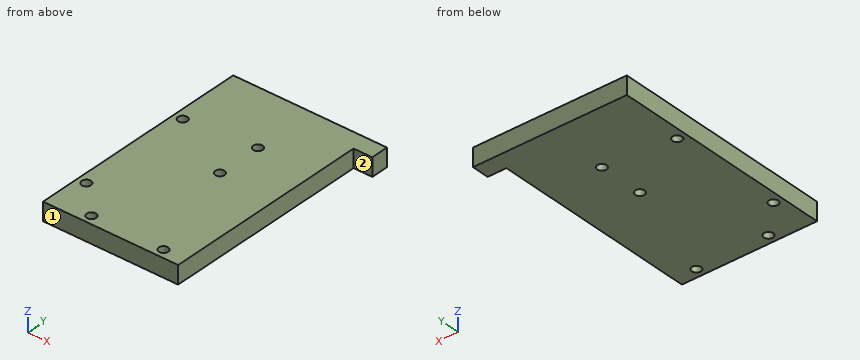
```python
from build123d import *

# Parameters (mm, degrees)
SZKIC1_W                    = 51
SZKIC1_H                    = 75
DODANIE_WYCI_GNI_CIE1_DEPTH = 6
SZKIC3_R                    = 1.55
WYTNIJ_WYCI_GNI_CIE1_DEPTH  = 99.368039697
SZKIC5_R                    = 1.55
WYTNIJ_WYCI_GNI_CIE2_DEPTH  = 6
SZKIC6_W                    = 6.4
SZKIC6_H                    = 69.4
WYTNIJ_WYCI_GNI_CIE3_DEPTH  = 10


with BuildPart() as part:
    # Szkic1 → Dodanie-wyciągnięcie1 (new body)
    with BuildSketch(Plane.XY):
        with Locations((29.991181586, 43.5)):
            Rectangle(SZKIC1_W, SZKIC1_H)
    extrude(amount=DODANIE_WYCI_GNI_CIE1_DEPTH)

    # Szkic3 → Wytnij-wyciągnięcie1 (cut, through all)
    with BuildSketch(Plane(origin=(0, 0, 0), x_dir=(-1, 0, 0), z_dir=(0, 0, -1))):
        with Locations((-18.041181586, 9)):
            Circle(SZKIC3_R)
        with Locations((-41.941181586, 9)):
            Circle(SZKIC3_R)
        with Locations((-7.491181586, 19.55)):
            Circle(SZKIC3_R)
        with Locations((-7.491181586, 57.55)):
            Circle(SZKIC3_R)
    extrude(amount=-WYTNIJ_WYCI_GNI_CIE1_DEPTH, mode=Mode.SUBTRACT)

    # Szkic5 → Wytnij-wyciągnięcie2 (cut)
    with BuildSketch(Plane(origin=(0, 0, 0), x_dir=(-1, 0, 0), z_dir=(0, 0, -1))):
        with Locations((-30.491181586, 59.871958533)):
            Circle(SZKIC5_R)
        with Locations((-30.491181586, 44.871958533)):
            Circle(SZKIC5_R)
    extrude(amount=-WYTNIJ_WYCI_GNI_CIE2_DEPTH, mode=Mode.SUBTRACT)

    # Szkic6 → Wytnij-wyciągnięcie3 (cut)
    with BuildSketch(Plane(origin=(0, 0, 0), x_dir=(-1, 0, 0), z_dir=(0, 0, -1))):
        with Locations((-52.491181586, 40.5)):
            Rectangle(SZKIC6_W, SZKIC6_H)
    extrude(amount=-WYTNIJ_WYCI_GNI_CIE3_DEPTH, mode=Mode.SUBTRACT)


solid = part.part
```
Geometry check sheet. Reference: the model listing, model coordinates, mm. Face numbers are marked on the shaded views. A direction names the side the tool comes from. Give positions to 0.01 mm unless a question says otherwise; leave off trailing zeros. Write each loop counter-clockwise with the first axis right and the second up, starting at its lowest first coordinate (ties: lowest second). Pieces come first, ordered by that corner, then holes. Notation, with made-up numbers: (87.25, -32) -> (125.25, -32) arc R28 cw to (125.25, -7) -> close; hole circle Ø4 at (55.25, 42). An arc over 180 degrees is marked (long way). One line per question, with ' | ' between items.
Item 1: Depth check by flat-ended pin: pin 1 (2.5 mm diameter, centred on x = 7.49, y = 19.55, fed in from -Z); pin 2 (1.8 mm diameter, centred on x = 52.5, z = 3, fed in from -Y); pin 3 (1.5 mm diameter, centred on y = 65, z = 4.5, fed in from +X). Enter the tip coordinate at first touch or a pass-through.
Determined:
pin 1: through | pin 2: y = 75.2 | pin 3: x = 49.29
Item 2: Scan lines: line 1 along X through (y, z) = (56.5, 3.75); line 2 along X through (y, z) = (73, 3.6); line 3 along Y through (x, z) = (41, 1.25). Record each from-to range of solid material in increasing order.
Determined:
line 1: 4.49 to 6.35, 8.63 to 49.29 | line 2: 4.49 to 49.29 | line 3: 6 to 7.77, 10.23 to 81
Item 3: Sectioned sample at A-A, the plane y = 9. Record the boundary of the cut face in (x, z).
Determined:
outline: (4.49, 0) -> (16.49, 0) -> (16.49, 6) -> (4.49, 6) -> close; (19.59, 0) -> (40.39, 0) -> (40.39, 6) -> (19.59, 6) -> close; (43.49, 0) -> (49.29, 0) -> (49.29, 6) -> (43.49, 6) -> close
Item 4: Sectioned sample at B-B, the plane y = 19.55. Record the boundary of the cut face in (x, z).
Determined:
outline: (4.49, 0) -> (5.94, 0) -> (5.94, 6) -> (4.49, 6) -> close; (9.04, 0) -> (49.29, 0) -> (49.29, 6) -> (9.04, 6) -> close
Item 5: Sectioned sample at C-C, the plane x = 42.5. Record the boundary of the cut face in (y, z), plus the area to 3 significant figures.
Determined:
outline: (6, 0) -> (7.55, 0) -> (7.55, 6) -> (6, 6) -> close; (10.45, 0) -> (81, 0) -> (81, 6) -> (10.45, 6) -> close | area: 433 mm^2
Item 6: Sectioned sample at D-D, the plane z = 4.35. Record the boundary of the cut face in (x, y), plus the area to 3 significant figures.
Determined:
outline: (4.49, 6) -> (49.29, 6) -> (49.29, 75.2) -> (55.49, 75.2) -> (55.49, 81) -> (4.49, 81) -> close; hole circle Ø3.1 at (7.49, 19.55); hole circle Ø3.1 at (7.49, 57.55); hole circle Ø3.1 at (18.04, 9); hole circle Ø3.1 at (30.49, 44.87); hole circle Ø3.1 at (30.49, 59.87); hole circle Ø3.1 at (41.94, 9) | area: 3,350 mm^2
Item 7: Access from +Z, -Z, +X, -X, +Y, -Y to the whole of each face (thin tool, end or side, straight path). Record for the marked faces 1 and 2.
Determined:
face 1: +Z, -Z, +X, -X, -Y | face 2: +Z, -Z, +X, -Y
